Input: part model. Units: mm. Frame: model coordinates. A direction names the side the tool comes from. Coordinates: 2 decimals unless noted, no trailing zeros. Loops run counter-clockwise (first coordinate to the right, second up) from the corner with the lowest first, then second, coordinate; pieces in that order, holes last. Notation, with made-up numbers: (49, -24) - (83, -24) arc R22 ccw to (83, -13) - close; hole circle Ø3 at (62.25, 32.5). An arc over 180 degrees is marked (long way). Answer as CSV lines item,"result". Start each with the question number.
```python
from build123d import *


with BuildPart() as part:
    # Austragung1: sweep along a path in Skizze1
    with BuildLine(Plane(origin=(0, 0, 0), x_dir=(1, 0, 0), z_dir=(0, 1, 0))) as austragung1_path:
        Line((-69.654529262, -21.528063223), (-81.174051866, -5.393202266))
        ThreePointArc((-81.174051866, -5.393202266), (-84.623968891, 9.520303277), (-76.517987713, 22.5052039))
        Line((-76.517987713, 22.5052039), (-74.310593415, 24.081178344))
        ThreePointArc((-74.310593415, 24.081178344), (-68.149421773, 31.204819131), (-65.931764421, 40.358413503))
        Line((-65.931764421, 40.358413503), (-65.931764421, 42.300814045))
        ThreePointArc((-65.931764421, 42.300814045), (-64.562830296, 49.572910331), (-60.643425983, 55.849504539))
        ThreePointArc((-60.643425983, 55.849504539), (0, 82.442660512), (60.643425983, 55.849504539))
        ThreePointArc((60.643425983, 55.849504539), (64.562830296, 49.572910331), (65.931764421, 42.300814045))
        Line((65.931764421, 42.300814045), (65.931764421, -42.300814045))
        ThreePointArc((65.931764421, -42.300814045), (64.562830296, -49.572910331), (60.643425983, -55.849504539))
        ThreePointArc((60.643425983, -55.849504539), (0, -82.442660512), (-60.643425983, -55.849504539))
        ThreePointArc((-60.643425983, -55.849504539), (-64.562830296, -49.572910331), (-65.931764421, -42.300814045))
        Line((-65.931764421, -42.300814045), (-65.931764421, -33.149234229))
        ThreePointArc((-65.931764421, -33.149234229), (-66.885180696, -27.04778781), (-69.654529262, -21.528063223))
    # Skizze2 → Austragung1 (sweep)
    with BuildSketch(Plane(origin=(0, 0, 0), x_dir=(0, 0, -1), z_dir=(1, 0, 0))):
        with BuildLine():
            Line((-82.442660512, 3.114282512), (-86.384630622, 3.114282512))
            Line((-86.384630622, 3.114282512), (-85.556943024, 0))
            ThreePointArc((-85.556943024, 0), (-80.240530229, -2.202130283), (-82.442660512, 3.114282512))
        make_face()
    sweep(path=austragung1_path.line)


solid = part.part
```
Item 1: Material intervals for probe 1 along X at (y, z) = (2.5, -45.5); probe 2 along X at (y, z) = (-2.5, 14); probe 3 along Z at (x, y) = (48.5, -1.75), sorted ascending.
Item 2: Section query A-A, the plane y = 1.5. Output: boundary loops of the cut face in (x, z), and give its area (3 significant figures).
Item 3: Draft query along X for faces 3 (the flat face through (-72, 3.114, 19)), 4 (the cylindrical face through (-74.078, -2.128, -21.454)), 5 (the conical face through (-71.332, 1.535, -32.72)), 6 (the cylindrical face through (-73.645, -2.128, 12.027)). Return one class per face: pulls with the +X half, pulls with the -X half, needs draft (parallel to the pull), parting line crosses it, or undercut.
Item 4: Set-up query: faces 1 (the cylindrical face through (-63.66, -2.13, 37.66)), 2 (the flat face through (-78.37, 1.58, 15.4)). Return all of +Z, -Z, +X, -X, +Y, -Y with unobstructed straight access to the full face (end or side cutting, diameter ignored); none if empty.
Item 5: Contact query for flat-ended pins moving along their axis: P1, Ø1.5, axis at x = 23, y = 2.5, coming from the -Z side; P2, Ø3, axis at y = -2, z = 58.5, coming from the -X side; P3, Ø3, axis at x = -38, y = -0.5, coming from the +Z side. Output: stop coordinate, or through.
Response values:
1,probe 1,"x = -69.49 to -63.79, 63.79 to 69.49"
1,probe 2,"x = -77.31 to -72.75, 64.07 to 67.79"
1,probe 3,"z = -69.83 to -63.45, 63.45 to 69.83"
2,outline,"(-84.03, 7.43) arc R23.51 ccw to (-78.56, -25.36) - (-76.35, -26.94) arc R16.49 cw to (-69.44, -40.36) - (-69.44, -42.3) arc R23.51 ccw to (-63.23, -58.23) arc R85.96 ccw to (63.23, -58.23) arc R23.51 ccw to (69.44, -42.3) - (69.44, 42.3) arc R23.51 ccw to (63.23, 58.23) arc R85.96 ccw to (-63.23, 58.23) arc R23.51 ccw to (-69.44, 42.3) - (-69.44, 33.15) arc R16.49 cw to (-72.51, 23.57) - close; hole (-78.95, 3.81) arc R17.27 ccw to (-74.93, -20.28) - (-72.72, -21.86) arc R22.73 cw to (-63.2, -40.36) - (-63.2, -42.3) arc R17.27 ccw to (-58.64, -54) arc R79.71 ccw to (58.64, -54) arc R17.27 ccw to (63.2, -42.3) - (63.2, 42.3) arc R17.27 ccw to (58.64, 54) arc R79.71 ccw to (-58.64, 54) arc R17.27 ccw to (-63.2, 42.3) - (-63.2, 33.15) arc R22.73 cw to (-67.43, 19.94) - close"
2,area,"3,220 mm²"
3,face 3,"needs draft"
3,face 4,"undercut"
3,face 5,"pulls with the -X half"
3,face 6,"undercut"
4,face 1,"none"
4,face 2,"+Z, -X, -Y"
5,P1,"stops at z = -83.39"
5,P2,"stops at x = -63.26"
5,P3,"stops at z = 77.36"
